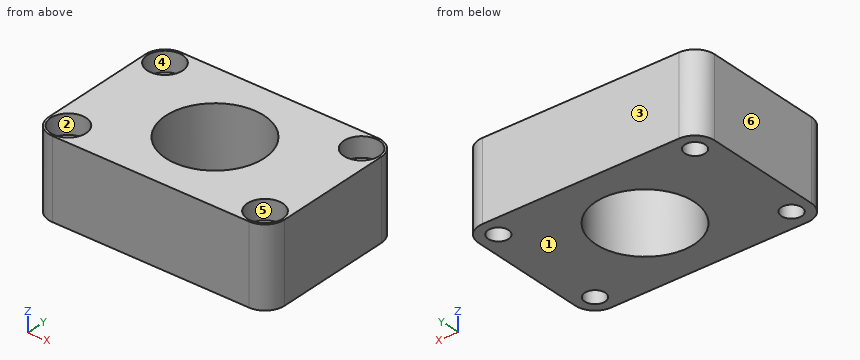
Autodesk Fusion 360 part; units mm, degrees
sketch "Sketch1" plane through (0, 0, 0) normal (0, 0, 1) x (1, 0, 0)
  line L0 (38.1, -25.4) -> (-38.1, -25.4)
  line L1 (-38.1, -25.4) -> (-38.1, 25.4)
  line L2 (-38.1, 25.4) -> (38.1, 25.4)
  line L3 (38.1, 25.4) -> (38.1, -25.4)
  line L4 (38.1, -25.4) -> (-38.1, 25.4) construction
  line L5 (-38.1, -25.4) -> (38.1, 25.4) construction
  circle A0 centre (0, 0) radius 15.875
  dimension "d1" = 76.2
  dimension "d2" = 50.8
  dimension "d3" = 31.75
extrude "Extrude1" add sketch "Sketch1" along normal blind 25.4
fillet "Fillet1" radius 6.35 4 edges at (38.1, 25.4, 12.7) (38.1, -25.4, 12.7) (-38.1, -25.4, 12.7) (-38.1, 25.4, 12.7)
sketch "Sketch2" plane through (0, 0, 25.4) normal (0, 0, 1) x (-1, 0, 0)
  circle A0 centre (0, 0) radius 15.875
  arc A1 (31.75, -25.4) -> (38.1, -19.05) centre (31.75, -19.05) ccw
  line L0 (38.1, -19.05) -> (38.1, 19.05)
  arc A2 (38.1, 19.05) -> (31.75, 25.4) centre (31.75, 19.05) ccw
  line L1 (31.75, 25.4) -> (-31.75, 25.4)
  arc A3 (-31.75, 25.4) -> (-38.1, 19.05) centre (-31.75, 19.05) ccw
  line L2 (-38.1, 19.05) -> (-38.1, -19.05)
  arc A4 (-38.1, -19.05) -> (-31.75, -25.4) centre (-31.75, -19.05) ccw
  line L3 (-31.75, -25.4) -> (31.75, -25.4)
  point P0 (31.75, -19.05)
  point P1 (-31.75, -19.05)
  point P2 (-31.75, 19.05)
  point P3 (31.75, 19.05)
hole "Hole1" at (-31.75, 19.05, 25.4) at (-31.75, -19.05, 25.4) at (31.75, -19.05, 25.4) at (31.75, 19.05, 25.4) direction (0, 0, -1) diameter 6.604 end through all counterbore diameter 11.43 counterbore depth 6.35
Verification items for the finished model (mm, model axes). Face numbers are marked on the shaded views. A direction names the side the tool comes from. Round coordinates to 2 decimals unless told otherwise and drop trailing zeros. Order: outer loops, then holes, each group sorted by start corner. A loop starts at its lowest first (then second) coordinate and runs counter-clockwise, first axis right, second up. Notation, with made-up numbers: (70.5, 15.25) -> (111.5, 15.25) arc R18 ccw to (111.5, 25.25) -> close; hole circle Ø4 at (73.5, 48.25). An arc over 180 degrees is marked (long way). Put each result on its own line as item: value.
1) Set-up check for the marked faces 1 and 2: record each of +Z, -Z, +X, -X, +Y, -Y from which the full face is reachable in a straight line by a thin tool's end or side.
Final values:
face 1: -Z, +X, -X, +Y, -Y
face 2: +Z
2) Section check D-D (y = -21.5). Record the cut outline in (x, z).
Final values:
outline: (-37.61, 0) -> (-33.96, 0) -> (-33.96, 19.05) -> (-36.91, 19.05) -> (-36.91, 25.4) -> (-37.61, 25.4) -> close; (-29.54, 0) -> (29.54, 0) -> (29.54, 19.05) -> (26.59, 19.05) -> (26.59, 25.4) -> (-26.59, 25.4) -> (-26.59, 19.05) -> (-29.54, 19.05) -> close; (33.96, 0) -> (37.61, 0) -> (37.61, 25.4) -> (36.91, 25.4) -> (36.91, 19.05) -> (33.96, 19.05) -> close
3) Section check A-A (y = 0). Record the cut outline in (x, z) (3 decimals).
Final values:
outline: (-38.1, 0) -> (-15.875, 0) -> (-15.875, 25.4) -> (-38.1, 25.4) -> close; (15.875, 0) -> (38.1, 0) -> (38.1, 25.4) -> (15.875, 25.4) -> close
4) Depth check by flat-ended pin: pin 1 (8.5 mm diameter, centred on x = -31.75, y = -19.05, fed in from +Z); pin 2 (5.5 mm diameter, centred on x = 31.75, y = 19.05, fed in from +Z). Enter the tip coordinate at first touch or a pass-through.
Final values:
pin 1: stops at z = 19.05
pin 2: passes through
5) Section check B-B (x = 0). Record the cut outline in (y, z) (3 decimals), then the cut area to 3 significant figures.
Final values:
outline: (-25.4, 0) -> (-15.875, 0) -> (-15.875, 25.4) -> (-25.4, 25.4) -> close; (15.875, 0) -> (25.4, 0) -> (25.4, 25.4) -> (15.875, 25.4) -> close
area: 484 mm^2
6) Material ranges on line 1 (X direction, y = 19.05, z = 22) (3 decimals); line 2 (Y direction, x = -31.75, z = 23) (3 decimals); line 3 (Y direction, x = -31.75, z = 5.25), recorded low to high.
Final values:
line 1: x = -38.1 to -37.465, -26.035 to 26.035, 37.465 to 38.1
line 2: y = -25.4 to -24.765, -13.335 to 13.335, 24.765 to 25.4
line 3: y = -25.4 to -22.35, -15.75 to 15.75, 22.35 to 25.4
7) Section check C-C (z = 20). Record the cut outline in (x, y) (3 decimals).
Final values:
outline: (-38.1, -19.05) arc R6.35 ccw to (-31.75, -25.4) -> (31.75, -25.4) arc R6.35 ccw to (38.1, -19.05) -> (38.1, 19.05) arc R6.35 ccw to (31.75, 25.4) -> (-31.75, 25.4) arc R6.35 ccw to (-38.1, 19.05) -> close; hole circle Ø11.43 at (-31.75, -19.05); hole circle Ø11.43 at (-31.75, 19.05); hole circle Ø31.75 at (0, 0); hole circle Ø11.43 at (31.75, -19.05); hole circle Ø11.43 at (31.75, 19.05)
8) Mould release check, pull along Y, two halves, no side actions. Record for the marked faces 3, 4, 5 and 6: +Y half, -Y half, draft (parallel to the pull), parting line (faces both ways), or undercut.
Final values:
face 3: +Y half
face 4: undercut
face 5: undercut
face 6: draft
